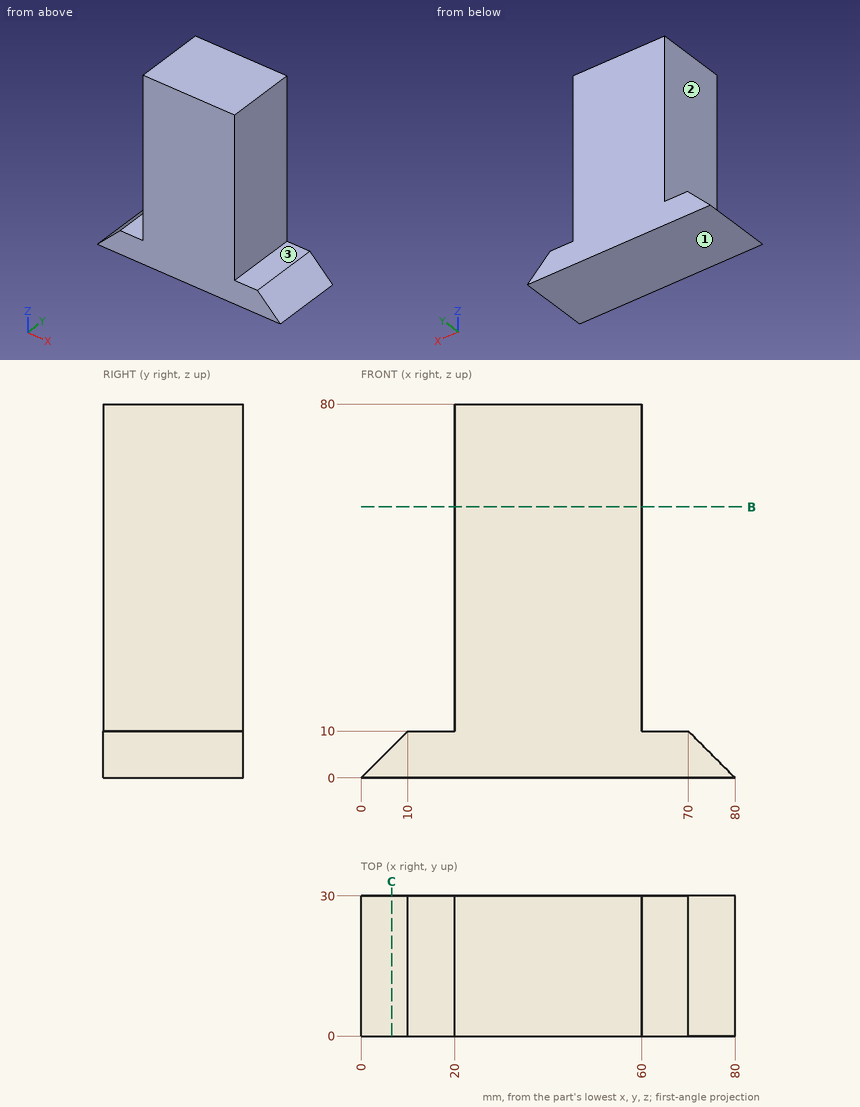
The figure shows three views and two pictorial views of one solid part (mm, origin at its lowest corner). Answer the questions. A direction names the side the tool comes from. Round coordinates to 2 decimals unless told otherwise and drop trailing zeros. Write each loop counter-clockwise with the first axis right and the second up, starting at its lowest first coordinate (ties: lowest second). Pieces come first, ordered by that corner, then holes. Notation, with made-up numbers: M -19.5,22 L 26.5,22 A20 ccw 26.5,49 Z; hole C 79,-14 d11. An arc over 180 degrees is marked long. Use a Markdown table: item, result.
1) The part is cut by section C-C on x = 6.5. Give the vertices of the cut face in (y, z), plus the area to 3 significant figures.
Taken from the geometry:
| item | result |
|---|---|
| outline | M 0,0 L 30,0 L 30,6.5 L 0,6.5 Z |
| area | 195 mm2 |
2) Flat-ended cylindrical pins translate along their axes: pin 1 (6 mm diameter, centred on y = 14, z = 46.5, fed in from -X); pin 2 (1 mm diameter, centred on y = 8, z = 10, fed in from +X); pin 3 (3 mm diameter, centred on x = 65, y = 19.5, fed in from +Z). Find the tip coordinate at first contact, or state that the pin passes through.
Taken from the geometry:
| item | result |
|---|---|
| pin 1 | stops at x = 20 |
| pin 2 | stops at x = 70.5 |
| pin 3 | stops at z = 10 |
3) Which of the six approach directions +Z, -Z, +X, -X, +Y, -Y give full straight-line access (tool end or side, diameter ignored) to the marked faces 1, 2 and 3?
Taken from the geometry:
| item | result |
|---|---|
| face 1 | -Z, +X, -X, +Y, -Y |
| face 2 | +Z, -X, +Y, -Y |
| face 3 | +Z, +X, +Y, -Y |
4) The part is cut by section B-B on z = 58. Give the vertices of the cut face in (x, y), plus the area to 3 significant figures.
Taken from the geometry:
| item | result |
|---|---|
| outline | M 20,0 L 60,0 L 60,30 L 20,30 Z |
| area | 1,200 mm2 |
5) Consider line 1 (X direction, y = 17, z = 48); line 2 (Z direction, x = 64, y = 12); line 3 (Z direction, x = 71, y = 22.5). Determine where each line is inside the solid, lowest interval first. Write a range as [from, to].
Taken from the geometry:
| item | result |
|---|---|
| line 1 | x = [20, 60] |
| line 2 | z = [0, 10] |
| line 3 | z = [0, 9] |
